Source: CAD feature listing. Evaluate the final solid. Frame: model axes, mm. Face numbers are marked on the shaded views. Round coordinates to 2 decimals unless told otherwise and drop trailing zeros. Loops run counter-clockwise (first coordinate to the right, second up) from the corner with the lowest first, then second, coordinate; pieces in that order, holes last. Notation, with made-up numbers: (-24, 76) -> (-16, 76) arc R22 ccw to (-16, 113) -> close; hole circle Ø5 at (74.25, 17.5). An arc over 180 degrees is marked (long way). Put each result on its own line as item: value. Start each with the question number.
1. Contact query for flat-ended pins moving along their axis: pin 1 (6 mm diameter, centred on x = 5, z = 8.5, fed in from +Y); pin 2 (1.5 mm diameter, centred on x = 6, z = 22.5, fed in from -Y); pin 3 (5 mm diameter, centred on x = 2, y = 2, fed in from +Z). Output: stop coordinate, or through.
2. Draft query along X for the marked faces 1 and 2. Return one class per face: pulls with the +X half, pulls with the -X half, needs draft (parallel to the pull), parting line crosses it, or undercut.
3. Cut plane D-D (x = -8.25). Return the cut outline in (y, z).
4. Material intervals for L1, parallel to Z at x = 1.75, y = -7; L2, parallel to X at y = 3.25, z = 22.75; L3, parallel to X at y = 2.75, z = 15, sorted ascending.
5. Cut plane A-A (x = -0.75). Return the cut outline in (y, z) (1 decimal).
6. Cut plane B-B (z = 4.25). Return the cut outline in (x, y).
7. Cut plane C-C (y = -6). Return the cut outline in (x, z).
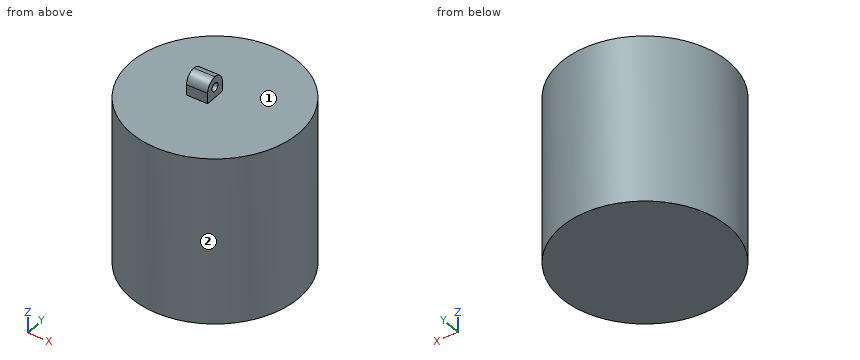
```python
from build123d import *

# Parameters (mm, degrees)
SKETCH2_R           = 12.7
BOSS_EXTRUDE1_DEPTH = 25.4
SKETCH3_W           = 3.175
SKETCH3_H           = 3.175
BOSS_EXTRUDE2_DEPTH = 3.175
CUT_EXTRUDE1_START  = -3.175
CUT_EXTRUDE1_DEPTH  = 3.175
SKETCH6_R           = 0.635
CUT_EXTRUDE2_DEPTH  = 2.54


# Read off the part's stored shape, not the designer's step: Cut-Extrude1
with BuildPart() as part:
    # Sketch2 → Boss-Extrude1 (new body)
    with BuildSketch(Plane.XY):
        Circle(SKETCH2_R)
    extrude(amount=BOSS_EXTRUDE1_DEPTH)

    # Sketch3 → Boss-Extrude2 (add)
    with BuildSketch(Plane.XY.offset(25.4)):
        with Locations((-1.5875, 0)):
            Rectangle(SKETCH3_W, SKETCH3_H)
    extrude(amount=BOSS_EXTRUDE2_DEPTH)

    # Cut-Extrude1 outline → Cut-Extrude1 (cut)
    with BuildSketch(Plane.ZY.offset(3.175).offset(CUT_EXTRUDE1_START)):
        with BuildLine():
            Line((28.575, 1.5875), (26.9875, 1.5875))
            ThreePointArc((26.9875, 1.5875), (28.110032015, 1.122532015), (28.575, 0))
            Line((28.575, 0), (28.575, 1.5875))
        make_face()
        with BuildLine():
            Line((28.575, -1.5875), (28.575, 0))
            ThreePointArc((28.575, 0), (28.110032015, -1.122532015), (26.9875, -1.5875))
            Line((26.9875, -1.5875), (28.575, -1.5875))
        make_face()
    extrude(amount=CUT_EXTRUDE1_DEPTH, mode=Mode.SUBTRACT)

    # Sketch6 → Cut-Extrude2 (cut)
    with BuildSketch(Plane(origin=(0, 0, 0), x_dir=(0, 0, -1), z_dir=(1, 0, 0))):
        with Locations((-26.9875, 0)):
            Circle(SKETCH6_R)
    extrude(amount=-CUT_EXTRUDE2_DEPTH, mode=Mode.SUBTRACT)


solid = part.part
```
Solution:
1. pin 1: stops at y = 12.54
1. pin 2: stops at y = -11.56
1. pin 3: stops at z = 28.49
2. face 1: needs draft
2. face 2: parting line crosses it
3. outline: (-9.66, 0) -> (9.66, 0) -> (9.66, 25.4) -> (-9.66, 25.4) -> close
4. L1: z = 0 to 25.4
4. L2: x = -12.28 to 12.28
4. L3: x = -12.4 to 12.4
5. outline: (-12.7, 0) -> (12.7, 0) -> (12.7, 25.4) -> (1.6, 25.4) -> (1.6, 27) arc R1.6 ccw to (-1.6, 27) -> (-1.6, 25.4) -> (-12.7, 25.4) -> close; hole circle Ø1.3 at (0, 27)
6. outline: circle Ø25.4 at (0, 0)
7. outline: (-11.19, 0) -> (11.19, 0) -> (11.19, 25.4) -> (-11.19, 25.4) -> close
